```python
from build123d import *

# Parameters (mm, degrees)
F_1_2_0_5_DIAMETER_HOLE1_D   = 12.7
F_1_1_DIAMETER_HOLE1_D       = 25.4
F_1_8_0_125_DIAMETER_HOLE1_D = 3.175


with BuildPart() as part:
    # Sketch1 → Revolve1 (revolve)
    with BuildSketch(Plane.XY):
        Polygon((-32.9565, 6.35), (-32.9565, 3.81), (-36.5125, 3.81), (-36.5125, 6.35), (-50.8, 6.35), (-50.8, 0), (0, 0), (0, 6.35), align=None)
    revolve(axis=Axis((0, 0, 0), (0, 1, 0)))

    # 1/2 (0.5) Diameter Hole1 (through all)
    with Locations(Plane(origin=(0, 6.35, 0), x_dir=(1, 0, 0), z_dir=(0, 1, 0))):
        with Locations((0, 0)):
            Hole(F_1_2_0_5_DIAMETER_HOLE1_D / 2)

    # 1 (1) Diameter Hole1 (through all)
    with Locations(Plane(origin=(0, 6.35, 0), x_dir=(1, 0, 0), z_dir=(0, 1, 0))):
        with Locations((50.8, 0), (-50.8, 0)):
            Hole(F_1_1_DIAMETER_HOLE1_D / 2)

    # 1/8 (0.125) Diameter Hole1 (through all)
    with Locations(Plane(origin=(0, 6.35, 0), x_dir=(1, 0, 0), z_dir=(0, 1, 0))):
        with Locations((38.494829198, 22.225)):
            Hole(F_1_8_0_125_DIAMETER_HOLE1_D / 2)


solid = part.part
```
The model under review builds one solid part; all positions refer to its coordinate system, in mm. A direction names the side the tool comes from. Coordinates: 2 decimals unless noted, no trailing zeros. Order: outer loops, then holes, each group sorted by start corner. A loop starts at its lowest first (then second) coordinate and runs counter-clockwise, first axis right, second up. Notation, with made-up numbers: M 22,35.5 L 75,35.5 A10 cw 75,47.5 Z; hole C 9,-0.5 d8. An arc over 180 degrees is marked long. One line per question, with ' | ' between items.
(1) Add section A-A, the plane x = 0. Write out the cut boundary in (y, z), then the cut area to 3 significant figures.
Geometry results:
outline: M 0,-50.8 L 6.35,-50.8 L 6.35,-36.51 L 3.81,-36.51 L 3.81,-32.96 L 6.35,-32.96 L 6.35,-6.35 L 0,-6.35 Z; M 0,6.35 L 6.35,6.35 L 6.35,32.96 L 3.81,32.96 L 3.81,36.51 L 6.35,36.51 L 6.35,50.8 L 0,50.8 Z | area: 546 mm²
(2) Add section D-D, the plane y = 2.5. State how many separate pieces and enclosed holes the cut face has, then the cut area to 3 significant figures.
Geometry results:
separate pieces: 1 | enclosed holes: 2 | area: 7,490 mm²
(3) Machinability: for faces 1 (the face through (38.103, 3.131, 0.257)), 2 (the face through (-6, 3.81, 33)), which of the approach directions +Z, -Z, +X, -X, +Y, -Y give a long, thin tool a straight path to every point of the face, cutting with its end or side? Answer none if there is none.
Geometry results:
face 1: +X, +Y, -Y | face 2: +Y
(4) Add section C-C, the plane x = 19.5. Write out the cut boundary in (y, z), then the cut area to 3 significant figures.
Geometry results:
outline: M 0,-46.91 L 6.35,-46.91 L 6.35,-30.87 L 3.81,-30.87 L 3.81,-26.57 L 6.35,-26.57 L 6.35,26.57 L 3.81,26.57 L 3.81,30.87 L 6.35,30.87 L 6.35,46.91 L 0,46.91 Z | area: 574 mm²
(5) The part is to be moulded in two halves that separate along Z. For faces 3 (the face through (4.29, 5.062, 32.676)), 4 (the face through (-0.94, 3.13, 50.79)), 5 (the face through (14, 6.35, -34)), say which applies: +Z half, -Z half, draft (parallel to the pull), parting line (faces both ways), or undercut.
Geometry results:
face 3: undercut | face 4: +Z half | face 5: draft
(6) Insertion check: pin 1 (8 mm diameter, centred on x = -38.5, z = 40, fed in from -Y); pin 2 (2 mm diameter, centred on x = 31, y = 3, fed in from +Z); pin 3 (1.5 mm diameter, centred on y = 5, z = -5, fed in from -X); pin 4 (1.5 mm diameter, centred on y = 3, z = -39.5, fed in from -X). Each pin has a flat end and moves straight along its axis. Give the tip position at first contact, or say it passes through.
Geometry results:
pin 1: passes through | pin 2: stops at z = 41 | pin 3: stops at x = -39.48 | pin 4: stops at x = -32.85
(7) For probe 1 along Z at (x, y) = (0, 5.4); probe 2 along Z at (x, y) = (20, 4.5); probe 3 along Z at (x, y) = (23.5, 4.25), list the stretches that pass through material, from the lowest coordinate up. Write a range as from..to.
Geometry results:
probe 1: z = -50.8..-36.51, -32.96..-6.35, 6.35..32.96, 36.51..50.8 | probe 2: z = -46.7..-30.55, -26.19..26.19, 30.55..46.7 | probe 3: z = -45.04..-27.94, -23.11..23.11, 27.94..45.04
(8) Add section B-B, the plane z = 0. Write out the cut boundary in (x, y).
Geometry results:
outline: M -38.1,0 L -6.35,0 L -6.35,6.35 L -32.96,6.35 L -32.96,3.81 L -36.51,3.81 L -36.51,6.35 L -38.1,6.35 Z; M 6.35,0 L 38.1,0 L 38.1,6.35 L 36.51,6.35 L 36.51,3.81 L 32.96,3.81 L 32.96,6.35 L 6.35,6.35 Z
